CAD build for the part. Positions are in the model's coordinates, mm. Face numbers are marked on the shaded views. A direction names the side the tool comes from. Round coordinates to 2 decimals unless told otherwise and drop trailing zeros. Loops run counter-clockwise (first coordinate to the right, second up) from the corner with the lowest first, then second, coordinate; pieces in that order, holes last.
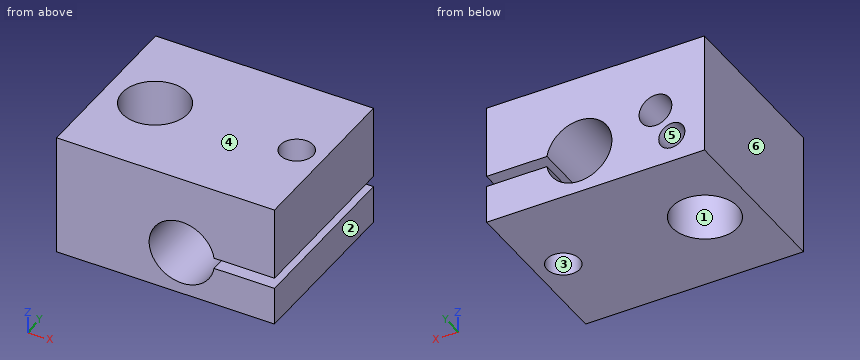
```python
from build123d import *

# Parameters (mm, degrees)
F0_W      = 20
F0_H      = 16
F1_DEPTH  = 11.2
F3_D      = 6
F4_D      = 3
F6_D      = 6
F7_D      = 3
F7_DEPTH  = 4
F7_TIP    = 0.9012909285
F8_D      = 2.4
F8_DEPTH  = 4
F8_TIP    = 0.7210327428
F9_W      = 12
F9_H      = 1
F10_DEPTH = 25


with BuildPart() as f1:
    # F0 (on Top) → F1 (new body)
    with BuildSketch(Plane.XY):
        Rectangle(F0_W, F0_H)
    extrude(amount=F1_DEPTH)

    # F3 (through all)
    with Locations(Plane.XY.offset(11.2)):
        with Locations((-5.5, 0)):
            Hole(F3_D / 2)

    # F4 (through all)
    with Locations(Plane.XY.offset(11.2)):
        with Locations((7.5, 0)):
            Hole(F4_D / 2)

    # F6 (through all)
    with Locations(Plane(origin=(0, 8, 0), x_dir=(-1, 0, 0), z_dir=(0, 1, 0))):
        with Locations((-1.5, 4)):
            Hole(F6_D / 2)

    # F7
    with Locations(Plane(origin=(0, 8, 0), x_dir=(-1, 0, 0), z_dir=(0, 1, 0))):
        with Locations((5.5, 5.5)):
            Hole(F7_D / 2, depth=F7_DEPTH)
            with Locations((0, 0, -(F7_DEPTH + F7_TIP / 2))):  # 118° drill point
                Cone(0, F7_D / 2, F7_TIP, mode=Mode.SUBTRACT)

    # F8
    with Locations(Plane(origin=(0, 8, 0), x_dir=(-1, 0, 0), z_dir=(0, 1, 0))):
        with Locations((7, 2.5)):
            Hole(F8_D / 2, depth=F8_DEPTH)
            with Locations((0, 0, -(F8_DEPTH + F8_TIP / 2))):  # 118° drill point
                Cone(0, F8_D / 2, F8_TIP, mode=Mode.SUBTRACT)

    # F9 (on face) → F10 (cut)
    with BuildSketch(Plane(origin=(0, 8, 0), x_dir=(-1, 0, 0), z_dir=(0, 1, 0))):
        with Locations((-10, 4)):
            Rectangle(F9_W, F9_H)
    extrude(amount=-F10_DEPTH, mode=Mode.SUBTRACT)


solid = f1.part
```
Item 1: Probe line 1 (Y direction, x = 7.5, z = 1); line 2 (Z direction, x = 9.25, y = 5.75); line 3 (X direction, y = 1.25, z = 6.25). List the from-to ranges inside material, lowest first.
Answers follow:
line 1: y = -8 to -1.5, 1.5 to 8
line 2: z = 0 to 3.5, 4.5 to 11.2
line 3: x = -10 to -8.23, -2.77 to -0.48, 3.48 to 6.67, 8.33 to 10
Item 2: Two-plate mould, pull along X, no slides. Class the marked faces 1, 2, 3 and 4: released by +X, released by -X, zero draft, split by the parting line, or undercut.
Answers follow:
face 1: undercut
face 2: released by +X
face 3: undercut
face 4: zero draft
Item 3: Cut at B-B, the plane x = 7.5. Give the cut face in (y, z), plus the area to 3 significant figures.
Answers follow:
outline: (-8, 0) - (-1.5, 0) - (-1.5, 3.5) - (-8, 3.5) - close; (-8, 4.5) - (-1.5, 4.5) - (-1.5, 11.2) - (-8, 11.2) - close; (1.5, 0) - (8, 0) - (8, 3.5) - (1.5, 3.5) - close; (1.5, 4.5) - (8, 4.5) - (8, 11.2) - (1.5, 11.2) - close
area: 133 mm2
Item 4: Cut at A-A, the plane y = 4.75. Give the cut face in (x, z).
Answers follow:
outline: (-10, 0) - (10, 0) - (10, 3.5) - (4.46, 3.5) arc R3 cw (long way) to (4.46, 4.5) - (10, 4.5) - (10, 11.2) - (-10, 11.2) - close; hole circle Ø2.4 at (-7, 2.5); hole circle Ø3 at (-5.5, 5.5)
Item 5: Cut at C-C, the plane z = 9.25. Give the cut face in (x, y), plus the area to 3 significant figures.
Answers follow:
outline: (-10, -8) - (10, -8) - (10, 8) - (-10, 8) - close; hole circle Ø6 at (-5.5, 0); hole circle Ø3 at (7.5, 0)
area: 285 mm2
Item 6: Cut at D-D, the plane x = 1.75. Give the cut face in (y, z).
Answers follow:
outline: (-8, 0) - (8, 0) - (8, 1.01) - (-8, 1.01) - close; (-8, 6.99) - (8, 6.99) - (8, 11.2) - (-8, 11.2) - close
Item 7: Flat gauge pins, fed straight in: P1, Ø3, axis at x = 2.5, z = 3, coming from the -Y side; P2, Ø2.5, axis at x = -5.5, z = 5.5, coming from the +Y side. Where does each tip first touch, or does it go through?
Answers follow:
P1: passes through
P2: stops at y = 3.85
Item 8: 3-axis set-ups, long thin cutter, end or side, ignore diameter. For the marked faces 5 and 6: which of +Z, -Z, +X, -X, +Y, -Y reach the whole face in a straight line?
Answers follow:
face 5: +Y
face 6: +Z, -Z, -X, +Y, -Y
